from build123d import *

# Parameters (mm, degrees)
SKETCH1_R           = 9
BOSS_EXTRUDE1_DEPTH = 50
SKETCH2_R           = 6
BOSS_EXTRUDE2_DEPTH = 15
BOSS_EXTRUDE3_START = 15
SKETCH3_R           = 6
BOSS_EXTRUDE3_DEPTH = 15
FILLET1_R           = 1
FILLET2_R           = 1


with BuildPart() as part:
    # Sketch1 → Boss-Extrude1 (new body)
    with BuildSketch(Plane(origin=(0, 0, 0), x_dir=(0, 0, -1), z_dir=(1, 0, 0))):
        Circle(SKETCH1_R)
    extrude(amount=BOSS_EXTRUDE1_DEPTH)

    # Sketch2 → Boss-Extrude2 (add)
    with BuildSketch(Plane(origin=(50, 0, 0), x_dir=(0, 0, -1), z_dir=(1, 0, 0))):
        Circle(SKETCH2_R)
    extrude(amount=BOSS_EXTRUDE2_DEPTH)

    # Sketch3 → Boss-Extrude3 (add)
    with BuildSketch(Plane.ZY.offset(BOSS_EXTRUDE3_START)):
        with Locations(Location((0, 0, 0), (0, 0, 180))):
            Circle(SKETCH3_R)
    extrude(amount=-BOSS_EXTRUDE3_DEPTH)

    # Fillet1
    fillet1_edges = [part.edges().sort_by_distance(p)[0] for p in [
        (-15, 0, 6),
    ]]
    fillet(fillet1_edges, radius=FILLET1_R)

    # Fillet2
    fillet2_edges = [part.edges().sort_by_distance(p)[0] for p in [
        (65, 0, 6),
    ]]
    fillet(fillet2_edges, radius=FILLET2_R)


solid = part.part
Model file for the job. Use its own axes, mm. A direction names the side the tool comes from. Give positions to 0.01 mm unless a question says otherwise; leave off trailing zeros. Order: outer loops, then holes, each group sorted by start corner. A loop starts at its lowest first (then second) coordinate and runs counter-clockwise, first axis right, second up. Notation, with made-up numbers: M 64.25,61.25 L 113.25,61.25 A29 cw 113.25,91.25 Z; hole C 43,-21.75 d1. An arc over 180 degrees is marked long. Put each result on its own line as item: value. Start each with the question number.
(1) Band-saw the part on D-D on x = 58. Give the cut face in (y, z), then the cut area to 3 significant figures.
(2) Band-saw the part on C-C on x = 47.5. Give the cut face in (y, z), then the cut area to 3 significant figures.
(3) Pin check, flat tips, straight feed: pin 1 Ø1 at (y, z) = (5, 5.5) entering from -X; pin 2 Ø1.5 at (x, z) = (24.5, 2.5) entering from +Y; pin 3 Ø2 at (x, z) = (-6, -1.5) entering from -Y. Stop position of each tip, or through.
(4) Tool access for faces 1 (the face through (57, 0, 6)), 2 (the face through (-7.098, -1.802, -5.723)), 3 (the face through (24.65, 8.923, 1.172)): list every direction of +Z, -Z, +X, -X, +Y, -Y with a clear straight run to the whole face (end or side of a thin tool).
(5) Drill centre lines: L1, parallel to X at y = -6.5, z = -3.25; L2, parallel to Y at x = 40, z = 0.75; L3, parallel to Z at x = 41.5, y = -7.5. Where is each one in solid material? Low to high. Write a range as [from, to].
(6) Band-saw the part on A-A on y = 0. Give the cut face in (x, z), then the cut area to 3 significant figures.
Results below:
1. outline: C 0,0 d12
1. area: 113 mm2
2. outline: C 0,0 d18
2. area: 254 mm2
3. pin 1: stops at x = 0
3. pin 2: stops at y = 8.83
3. pin 3: stops at y = -5.98
4. face 1: +X
4. face 2: -X
4. face 3: +X, -X
5. L1: x = [0, 50]
5. L2: y = [-8.97, 8.97]
5. L3: z = [-4.97, 4.97]
6. outline: M -15,-5 A1 ccw -14,-6 L 0,-6 L 0,-9 L 50,-9 L 50,-6 L 64,-6 A1 ccw 65,-5 L 65,5 A1 ccw 64,6 L 50,6 L 50,9 L 0,9 L 0,6 L -14,6 A1 ccw -15,5 Z
6. area: 1,260 mm2
